from build123d import *

# Parameters (mm, degrees)
F0_R     = 9.42624
F1_DEPTH = 213.868
F3_DEPTH = 50.8


with BuildPart() as f1:
    # F0 (on Right) → F1 (new body)
    with BuildSketch(Plane.YZ):
        Circle(F0_R)
    extrude(amount=F1_DEPTH)

    # F2 (on face) → F3 (join)
    with BuildSketch(Plane(origin=(0, 0, 0), x_dir=(0, -1, 0), z_dir=(-1, 0, 0))):
        Polygon((27.016499, 37.185021), (-27.016499, 37.185021), (-43.713614, -14.203414), (0, -45.963213), (43.713614, -14.203414), align=None)
    extrude(amount=-F3_DEPTH)


solid = f1.part
Part model, mm, in its own coordinate system. A direction names the side the tool comes from. Coordinates: 2 decimals unless noted, no trailing zeros. Order: outer loops, then holes, each group sorted by start corner. A loop starts at its lowest first (then second) coordinate and runs counter-clockwise, first axis right, second up.
(1) Probe L1, parallel to X at y = 38, z = -6.5; L2, parallel to Z at x = 39, y = -3; L3, parallel to Z at x = 16.5, y = 10.5. List the from-to ranges inside material, lowest first.
Check sheet entries:
L1: x = 0 to 50.8
L2: z = -43.78 to 37.19
L3: z = -38.33 to 37.19
(2) Tool access for faces 1 (the face through (50.8, -9, -4)), 2 (the face through (25.044, -21.551, -30.306)): list every direction of +Z, -Z, +X, -X, +Y, -Y with a clear straight run to the whole face (end or side of a thin tool).
Check sheet entries:
face 1: +X
face 2: -Z, +X, -X, -Y
(3) Pin check, flat tips, straight feed: pin 1 Ø3 at (x, z) = (174, -10) entering from +Y; pin 2 Ø12 at (y, z) = (13.5, -9) entering from +X; pin 3 Ø12 at (x, y) = (85.5, 2) entering from +Z. Stop position of each tip, or through.
Check sheet entries:
pin 1: stops at y = 4.07
pin 2: stops at x = 50.8
pin 3: stops at z = 9.43
(4) Slice it at C-C, the plane y = 23. Write the cut outline in (x, z).
Check sheet entries:
outline: (0, -29.25) - (50.8, -29.25) - (50.8, 37.19) - (0, 37.19) - close
(5) Slice it at D-D, the plane z = 21. Write the cut outline in (x, y), and give its area (3 significant figures).
Check sheet entries:
outline: (0, -32.28) - (50.8, -32.28) - (50.8, 32.28) - (0, 32.28) - close
area: 3,280 mm2
(6) Slice it at B-B, the plane x = 107. Write the cut outline in (y, z), and give its area (3 significant figures).
Check sheet entries:
outline: circle Ø18.85 at (0, 0)
area: 279 mm2
(7) Slice it at A-A, the plane z = 0. Write the cut outline in (x, y).
Check sheet entries:
outline: (0, -39.1) - (50.8, -39.1) - (50.8, -9.43) - (213.87, -9.43) - (213.87, 9.43) - (50.8, 9.43) - (50.8, 39.1) - (0, 39.1) - close
